CAD build for the part. Positions are in the model's coordinates, mm. Face numbers are marked on the shaded views. A direction names the side the tool comes from. Coordinates: 2 decimals unless noted, no trailing zeros. Order: outer loops, then holes, each group sorted by start corner. A loop starts at its lowest first (then second) coordinate and runs counter-clockwise, first axis right, second up. Notation, with made-up numbers: M -11,34.25 L -4,34.25 A23 ccw -4,62.25 Z; hole C 20.5,87.25 d11. An arc over 180 degrees is marked long. One line per item, written item: value.
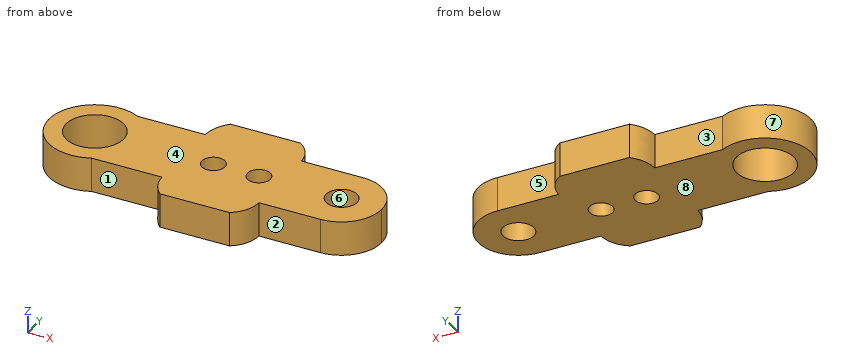
from build123d import *

# Parameters (mm, degrees)
SKETCH_3_R      = 2.5
SKETCH_3_R_2    = 1
SKETCH_3_R_3    = 1.35
EXTRUDE_2_DEPTH = 3


with BuildPart() as part:
    # 草图3 → 凸台-拉伸2 (new body)
    with BuildSketch(Plane.XY):
        with BuildLine():
            Line((21.499968123, 3.52141019), (16.156278552, 3.52141019))
            add(Edge.make_bspline(
                [(16.156278552, 3.52141019), (16.088160339, 5.051537173), (14.821900334, 5.873909505)],
                knots=[0, 0, 0, 1, 1, 1], degree=2))
            Line((14.821900334, 5.873909505), (8.771282217, 5.873909505))
            add(Edge.make_bspline(
                [(7.754778373, 3.595279655), (7.816403966, 4.944689103), (8.771282217, 5.873909505)],
                knots=[0, 0, 0, 1, 1, 1], degree=2))
            Line((7.754778373, 3.595279655), (1.868346732, 3.595279655))
            ThreePointArc((1.868346732, 3.595279655), (-3.997767344, 0.192060873), (1.627998751, -3.595279655))
            Line((1.627998751, -3.595279655), (7.754778373, -3.595279655))
            add(Edge.make_bspline(
                [(7.754778373, -3.595279655), (7.816403966, -4.944689103), (8.771282217, -5.873909505)],
                knots=[0, 0, 0, 1, 1, 1], degree=2))
            Line((8.771282217, -5.873909505), (14.821900334, -5.873909505))
            add(Edge.make_bspline(
                [(16.156278552, -3.52141019), (16.088160339, -5.051537173), (14.821900334, -5.873909505)],
                knots=[0, 0, 0, 1, 1, 1], degree=2))
            Line((16.156278552, -3.52141019), (21.499968123, -3.52141019))
            ThreePointArc((21.499968123, -3.52141019), (23.982399961, -2.488702667), (24.999902637, 0))
            ThreePointArc((24.999902637, 0), (23.982399961, 2.488702667), (21.499968123, 3.52141019))
        make_face()
        with Locations((0, 0.058433534)):
            Circle(SKETCH_3_R, mode=Mode.SUBTRACT)
        with Locations((10.35, 0)):
            Circle(SKETCH_3_R_2, mode=Mode.SUBTRACT)
        with Locations((14.31, 0)):
            Circle(SKETCH_3_R_2, mode=Mode.SUBTRACT)
        with Locations((21.499968123, 0.02141019)):
            Circle(SKETCH_3_R_3, mode=Mode.SUBTRACT)
    extrude(amount=EXTRUDE_2_DEPTH)


solid = part.part
Q1. Slice it at C-C (z = 2.3). Give the number of separate pieces and of enclosed holes in the cut face, plus the area to 3 significant figures.
Recorded:
separate pieces: 1
enclosed holes: 4
area: 203 mm^2
Q2. Slice it at D-D (x = 16.5). List the corners of the cut face in (y, z).
Recorded:
outline: M -3.52,0 L 3.52,0 L 3.52,3 L -3.52,3 Z
Q3. Slice it at B-B (x = 10.35). List the corners of the cut face in (y, z), plus the area to 3 significant figures.
Recorded:
outline: M -5.87,0 L -1,0 L -1,3 L -5.87,3 Z; M 1,0 L 5.87,0 L 5.87,3 L 1,3 Z
area: 29.2 mm^2
Q4. Slice it at A-A (x = 0). List the corners of the cut face in (y, z).
Recorded:
outline: M -3.94,0 L -2.44,0 L -2.44,3 L -3.94,3 Z; M 2.56,0 L 4.06,0 L 4.06,3 L 2.56,3 Z
Q5. Mould opens along Y. For the marked faces 6, 7 and 8 say: released by +Y, released by -Y, zero draft, split by the parting line, or undercut.
Recorded:
face 6: undercut
face 7: split by the parting line
face 8: zero draft
Q6. Which spindle directions (+Z, -Z, +X, -X, +Y, -Y) get a long thin tool onto all of the face, cutting with end or side? Do the marked faces 1, 2, 3, 4 and 5. Say none if no direction does.
Recorded:
face 1: +Z, -Z, -Y
face 2: +Z, -Z, +X, -Y
face 3: +Z, -Z, +Y
face 4: +Z, +X, -X, +Y, -Y
face 5: +Z, -Z, +X, +Y
Q7. Drill centre lines: line 1 along Y through (x, z) = (14.31, 2.2); line 2 along Y through (x, z) = (0, 0.9); line 3 along X through (y, z) = (0.25, 2.7). Where is each one in solid material? Low to high.
Recorded:
line 1: y = -5.87 to -1, 1 to 5.87
line 2: y = -3.94 to -2.44, 2.56 to 4.06
line 3: x = -4 to -2.49, 2.49 to 9.38, 11.32 to 13.34, 15.28 to 20.17, 22.83 to 24.99
Q8. Pin check, flat tips, straight feed: pin 1 Ø1.5 at (x, z) = (5, 1.5) entering from -Y; pin 2 Ø4 at (x, y) = (0, 0.06) entering from +Z. Stop position of each tip, or through.
Recorded:
pin 1: stops at y = -3.6
pin 2: passes through
